Here's how the part is built. I have some questions about the finished solid (model axes, mm). A direction names the side the tool comes from. Coordinates: 2 decimals unless noted, no trailing zeros. Write each loop counter-clockwise with the first axis right and the second up, starting at its lowest first coordinate (ties: lowest second). Pieces come first, ordered by that corner, then holes. Notation, with made-up numbers: (87, 42.25) -> (96, 42.25) arc R28 ccw to (96, 80.25) -> close; hole circle Ø11 at (-32.75, -13). An arc over 180 degrees is marked (long way). Use a Markdown table: item, result. Add a question column.
```python
from build123d import *

# Parameters (mm, degrees)
SKETCH_1_W           = 12.5
SKETCH_1_H           = 22.5
EXTRUDE_1_DEPTH      = 5
CUT_EXTRUDE_2_DEPTH  = 29.25
CUT_EXTRUDE_4_DEPTH  = 29.25
SKETCH_1_9_R         = 1.5
SKETCH_1_9_W         = 3
SKETCH_1_9_H         = 4.5
EXTRUDE_2_DEPTH      = 4
EXTRUDE_7_DEPTH      = 5
EXTRUDE_7_DEPTH_BACK = 4
SKETCH_1_11_W        = 18.5
SKETCH_1_11_H        = 20
CUT_EXTRUDE_5_DEPTH  = 53.961684263
CUT_EXTRUDE_START    = -9
CUT_EXTRUDE_7_DEPTH  = 9
CUT_EXTRUDE_8_DEPTH  = 11
CUT_EXTRUDE_START_2  = -2
SKETCH_10_R          = 1.5
CUT_EXTRUDE_9_DEPTH  = 2


with BuildPart() as part:
    # 草图1 → 凸台-拉伸1 (new body)
    with BuildSketch(Plane.XY):
        Polygon((-9.25, 11), (-37.5, 11), (-37.5, -1), (-9.25, -1), (-9.25, -16.3), (9.25, -16.3), (9.25, -1), (37.5, -1), (37.5, 11), (9.25, 11), (9.25, 16.3), (-9.25, 16.3), align=None)
        Rectangle(SKETCH_1_W, SKETCH_1_H, mode=Mode.SUBTRACT)
    extrude(amount=EXTRUDE_1_DEPTH)

    # 草图2 → 切除-拉伸2 (cut)
    with BuildSketch(Plane.ZY.offset(37.5)):
        Polygon((5, 7), (5, 3), (2, 1), (2, 9), align=None)
    extrude(amount=-CUT_EXTRUDE_2_DEPTH, mode=Mode.SUBTRACT)

    # 草图3 → 切除-拉伸4 (cut)
    with BuildSketch(Plane(origin=(37.5, 0, 0), x_dir=(0, 0, -1), z_dir=(1, 0, 0))):
        Polygon((-5, 7), (-5, 3), (-2, 1), (-2, 9), align=None)
    extrude(amount=-CUT_EXTRUDE_4_DEPTH, mode=Mode.SUBTRACT)

    # 草图1<9> → 凸台-拉伸2 (add)
    # profile 1 of 8: a face of its own
    with BuildSketch(Plane.XY):
        Polygon((-9.25, 11), (-6.25, 11), (-6.25, 11.25), (0, 11.25), (6.25, 11.25), (6.25, 11), (9.25, 11), (9.25, 16.3), (-9.25, 16.3), align=None)
        with Locations((0, 13.8)):
            Circle(SKETCH_1_9_R, mode=Mode.SUBTRACT)
    # profile 2 of 8: a face of its own
    with BuildSketch(Plane.XY):
        with Locations((-7.75, 8.75)):
            Rectangle(SKETCH_1_9_W, SKETCH_1_9_H)
    # profile 3 of 8: a face of its own
    with BuildSketch(Plane.XY):
        with Locations((7.75, 8.75)):
            Rectangle(SKETCH_1_9_W, SKETCH_1_9_H)
    # profile 4 of 8: a face of its own
    with BuildSketch(Plane.XY):
        Polygon((6.25, 5), (6.25, 3.5), (9.25, 3.5), (9.25, 6.5), (6.25, 6.5), align=None)
    # profile 5 of 8: a face of its own
    with BuildSketch(Plane.XY):
        with Locations((7.75, 1.25)):
            Rectangle(SKETCH_1_9_W, SKETCH_1_9_H)
    # profile 6 of 8: a face of its own
    with BuildSketch(Plane.XY):
        Polygon((6.25, -11.25), (-6.25, -11.25), (-6.25, -1), (-9.25, -1), (-9.25, -16.3), (9.25, -16.3), (9.25, -1), (6.25, -1), align=None)
        with Locations((0, -13.8)):
            Circle(SKETCH_1_9_R, mode=Mode.SUBTRACT)
    # profile 7 of 8: a face of its own
    with BuildSketch(Plane.XY):
        with Locations((-7.75, 1.25)):
            Rectangle(SKETCH_1_9_W, SKETCH_1_9_H)
    # profile 8 of 8: a face of its own
    with BuildSketch(Plane.XY):
        Polygon((-9.25, 3.5), (-6.25, 3.5), (-6.25, 4.999999998), (-6.25, 6.5), (-9.25, 6.5), align=None)
    extrude(amount=-EXTRUDE_2_DEPTH)

    # 草图1<11> → 凸台-拉伸7 (add, two sides: drawn at the far end of the back side and taken through both)
    with BuildSketch(Plane.XY.offset(-EXTRUDE_7_DEPTH_BACK)):
        with Locations((0, 26.3)):
            Rectangle(SKETCH_1_11_W, SKETCH_1_11_H)
    extrude(amount=EXTRUDE_7_DEPTH + EXTRUDE_7_DEPTH_BACK)

    # 草图6 → 切除-拉伸5 (cut, through all)
    with BuildSketch(Plane.XY.offset(5)):
        Polygon((9.25, 23.775), (9.25, 27.775), (4.25, 31.275), (4.25, 23.775), align=None)
        Polygon((9.25, 19.775), (9.25, 23.775), (4.25, 23.775), (4.25, 16.275), align=None)
    extrude(amount=-CUT_EXTRUDE_5_DEPTH, mode=Mode.SUBTRACT)

    # 草图6<4> → 切除-拉伸7 (cut)
    with BuildSketch(Plane.XY.offset(5).offset(CUT_EXTRUDE_START)):
        with BuildLine():
            ThreePointArc((-1.65, 23.775), (0, 22.125), (1.65, 23.775))
            Line((1.65, 23.775), (-1.65, 23.775))
        make_face()
        with BuildLine():
            Line((-1.65, 23.775), (1.65, 23.775))
            ThreePointArc((1.65, 23.775), (0, 25.425), (-1.65, 23.775))
        make_face()
        with BuildLine():
            ThreePointArc((-1.65, 23.775), (0, 22.125), (1.65, 23.775))
            Line((1.65, 23.775), (-1.65, 23.775))
        make_face()
        with BuildLine():
            Line((-1.65, 23.775), (1.65, 23.775))
            ThreePointArc((1.65, 23.775), (0, 25.425), (-1.65, 23.775))
        make_face()
    extrude(amount=CUT_EXTRUDE_7_DEPTH, mode=Mode.SUBTRACT)

    # 草图9 → 切除-拉伸8 (cut)
    with BuildSketch(Plane.ZY.offset(9.25)):
        with BuildLine():
            ThreePointArc((2.15, 23.77), (0.5, 25.42), (-1.15, 23.77))
            Line((-1.15, 23.77), (2.15, 23.77))
        make_face()
        with BuildLine():
            Line((2.15, 23.77), (-1.15, 23.77))
            ThreePointArc((-1.15, 23.77), (0.5, 22.12), (2.15, 23.77))
        make_face()
        with BuildLine():
            ThreePointArc((2.15, 23.77), (0.5, 25.42), (-1.15, 23.77))
            Line((-1.15, 23.77), (2.15, 23.77))
        make_face()
        with BuildLine():
            Line((2.15, 23.77), (-1.15, 23.77))
            ThreePointArc((-1.15, 23.77), (0.5, 22.12), (2.15, 23.77))
        make_face()
    extrude(amount=-CUT_EXTRUDE_8_DEPTH, mode=Mode.SUBTRACT)

    # 草图10 → 切除-拉伸9 (cut)
    with BuildSketch(Plane(origin=(0, 0, 0), x_dir=(-1, 0, 0), z_dir=(0, 0, -1)).offset(CUT_EXTRUDE_START_2)):
        with Locations(Location((0, 13.8, 0), (0, 0, 180))):
            Circle(SKETCH_10_R)
        with Locations(Location((0, -13.8, 0), (0, 0, 180))):
            Circle(SKETCH_10_R)
    extrude(amount=CUT_EXTRUDE_9_DEPTH, mode=Mode.SUBTRACT)


solid = part.part
```
Q1. Suppose I cut it at C-C, the plane z = 3.5. State how many separate pieces and enclosed holes the cut face has, and give its area (3 significant figures).
Q2. Suppose I cut it at A-A, the plane y = 8. Write out the boundary of the cut face in (x, z), and give its area (3 significant figures).
Q3. Thinking about a two-plate mould opening in X: for faces 1 (the flat face through (6.715, 18, 0.563)), 2 (the flat face through (8.25, 5, 3)), 3 (the flat face through (23, 5, 2)), which applies, released by +X, released by -X, zero draft, split by the parting line, or undercut?
Q4. Which directions (+Z, -Z, +X, -X, +Y, -Y) give clear straight access to the entire face, cutting with the end or side of a thin tool? Please do faces 4 (the flat face through (23, -1, 2)), 5 (the flat face through (6.785, 29.5, 0.563)), 6 (the flat face through (-8.25, 5, 3)), 7 (the flat face through (0, -14, 2)), 8 (the flat face through (-24, -1, 2)).
Q5. Suppose I cut it at B-B, the plane x = 27. Write out the boundary of the cut face in (y, z).
Q6. Suppose I cut it at D-D, the plane y = -13.8. Write out the boundary of the cut face in (x, z), and give its area (4 significant figures).
Q7. Will these pins go through, and if not, where does the flat tip stop? pin 1 (3.5 mm diameter, centred on x = -23.5, y = 5.5, fed in from -Z); pin 2 (3 mm diameter, centred on y = 12.5, z = -2, fed in from -X); pin 3 (2.5 mm diameter, centred on y = 5, z = 3.5, fed in from -X).
Q8. Please list where these lines run through material, in increasing order: line 1 (Y direction, x = 0, z = 0) (3 decimals); line 2 (Y direction, x = -2, z = 0.5); line 3 (X direction, y = -13.8, z = -0.3).
Answer key:
| question | item | result |
|---|---|---|
| 1 | separate pieces | 1 |
| 1 | enclosed holes | 2 |
| 1 | area | 953 mm^2 |
| 2 | outline | (-37.5, 0) -> (-9.25, 0) -> (-9.25, -4) -> (-6.25, -4) -> (-6.25, 5) -> (-37.5, 5) -> (-37.5, 3.5) -> (-8.25, 3.5) -> (-8.25, 2) -> (-37.5, 2) -> close; (6.25, -4) -> (9.25, -4) -> (9.25, 0) -> (37.5, 0) -> (37.5, 2) -> (8.25, 2) -> (8.25, 3.5) -> (37.5, 3.5) -> (37.5, 5) -> (6.25, 5) -> close |
| 2 | area | 249 mm^2 |
| 3 | face 1 | undercut |
| 3 | face 2 | released by +X |
| 3 | face 3 | zero draft |
| 4 | face 4 | +Z, -Z, +X, -Y |
| 4 | face 5 | +Z, -Z |
| 4 | face 6 | -X |
| 4 | face 7 | -Z |
| 4 | face 8 | +Z, -Z, -X, -Y |
| 5 | outline | (-1, 0) -> (11, 0) -> (11, 5) -> (7, 5) -> (9, 2) -> (1, 2) -> (3, 5) -> (-1, 5) -> close |
| 6 | outline | (-9.25, -4) -> (-1.5, -4) -> (-1.5, 2) -> (1.5, 2) -> (1.5, -4) -> (9.25, -4) -> (9.25, 5) -> (-9.25, 5) -> close |
| 6 | area | 148.5 mm^2 |
| 7 | pin 1 | stops at z = 0 |
| 7 | pin 2 | stops at x = -9.25 |
| 7 | pin 3 | stops at x = -8.25 |
| 8 | line 1 | y = -16.3 to -15.3, -12.3 to -11.25, 11.25 to 12.3, 15.3 to 22.125, 25.425 to 36.3 |
| 8 | line 2 | y = -16.3 to -11.25, 11.25 to 22.12, 25.42 to 36.3 |
| 8 | line 3 | x = -9.25 to -1.5, 1.5 to 9.25 |
